Source: CAD feature listing. Evaluate the final solid. Frame: model axes, mm. Face numbers are marked on the shaded views. A direction names the side the tool comes from. Round coordinates to 2 decimals unless told otherwise and drop trailing zeros. Loops run counter-clockwise (first coordinate to the right, second up) from the corner with the lowest first, then second, coordinate; pieces in that order, holes last. Notation, with made-up numbers: (71.25, 12) -> (120.25, 12) arc R20 cw to (120.25, 51) -> close; hole circle Ø9 at (66, 28.5). An arc over 180 degrees is marked (long way). Return JSON: item names as keys, results as strings. Group by question number.
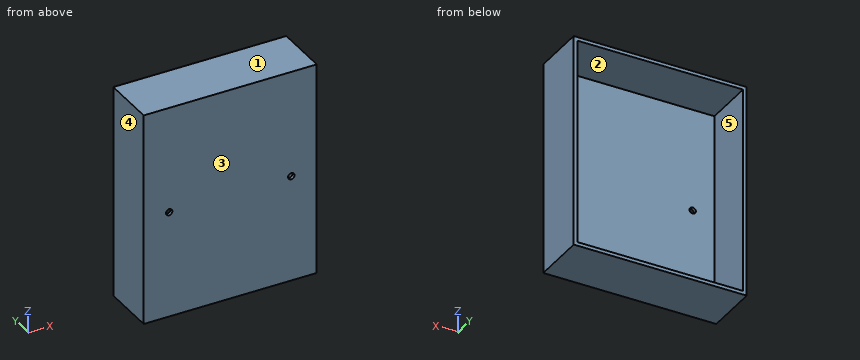
```python
from build123d import *

# Parameters (mm, degrees)
SKETCH1_W           = 61.2
SKETCH1_H           = 75.5
BOSS_EXTRUDE1_DEPTH = 19.15
SKETCH2_W           = 58.6
SKETCH2_H           = 72.89934915
CUT_EXTRUDE1_DEPTH  = 18
SKETCH3_R           = 1.125
CUT_EXTRUDE2_DEPTH  = 20


with BuildPart() as part:
    # Sketch1 → Boss-Extrude1 (new body)
    with BuildSketch(Plane(origin=(0, 0, 0), x_dir=(1, 0, 0), z_dir=(0, 1, 0))):
        Rectangle(SKETCH1_W, SKETCH1_H)
    extrude(amount=BOSS_EXTRUDE1_DEPTH)

    # Sketch2 → Cut-Extrude1 (cut)
    with BuildSketch(Plane(origin=(0, 19.15, 0), x_dir=(1, 0, 0), z_dir=(0, 1, 0))):
        Rectangle(SKETCH2_W, SKETCH2_H)
    extrude(amount=-CUT_EXTRUDE1_DEPTH, mode=Mode.SUBTRACT)

    # Sketch3 → Cut-Extrude2 (cut)
    with BuildSketch(Plane(origin=(0, 1.15, 0), x_dir=(1, 0, 0), z_dir=(0, 1, 0))):
        with Locations(Location((-21.6, 0, 0), (0, 0, 270))):
            Circle(SKETCH3_R)
        with Locations(Location((21.6, 0, 0), (0, 0, 270))):
            Circle(SKETCH3_R)
    extrude(amount=-CUT_EXTRUDE2_DEPTH, mode=Mode.SUBTRACT)


solid = part.part
```
(1) Cut plane B-B (z = 0). Return loops of the section in (x, y) (3 decimals).
(2) Pin query (flat end, axial travel): pin 1 (1 mm diameter, centred on x = -6, z = 28, fed in from +Y). Return the tip coordinate at first contact, or that it passes through.
(3) Mould query, pull axis X, two halves, no side actions, for the marked faces 3, 4 and 5. Classes: released by +X, released by -X, zero draft, split by the parting line, or undercut.
(4) Cut plane C-C (y = 11.5). Return loops of the section in (x, z), and give its area (3 significant figures).
(5) Cut plane A-A (x = -21.6). Return loops of the section in (y, z) (3 decimals), and give its area (3 significant figures).
(6) Set-up query: the marked faces 1 and 2. Return all of +Z, -Z, +X, -X, +Y, -Y with unobstructed straight access to the full face (end or side cutting, diameter ignored); none if empty.
(7) Cut plane D-D (z = -29). Return loops of the section in (x, y).
(8) Ray query, line 1 (X direction, y = 0.55, z = 0) (3 decimals); line 2 (Z direction, x = -5.5, y = 18); line 3 (X direction, y = 11.5, z = -0.5). Return the intervals inside material, ascending.
Answers follow:
{
 "1": {"outline": "(-30.6, 0) -> (-22.725, 0) -> (-22.725, 1.15) -> (-29.3, 1.15) -> (-29.3, 19.15) -> (-30.6, 19.15) -> close; (-20.475, 0) -> (20.475, 0) -> (20.475, 1.15) -> (-20.475, 1.15) -> close; (22.725, 0) -> (30.6, 0) -> (30.6, 19.15) -> (29.3, 19.15) -> (29.3, 1.15) -> (22.725, 1.15) -> close"},
 "2": {"pin 1": "y = 1.15"},
 "3": {"face 3": "zero draft", "face 4": "released by -X", "face 5": "undercut"},
 "4": {"outline": "(-30.6, -37.75) -> (30.6, -37.75) -> (30.6, 37.75) -> (-30.6, 37.75) -> close; hole (-29.3, -36.45) -> (29.3, -36.45) -> (29.3, 36.45) -> (-29.3, 36.45) -> close", "area": "349 mm^2"},
 "5": {"outline": "(0, -37.75) -> (19.15, -37.75) -> (19.15, -36.45) -> (1.15, -36.45) -> (1.15, -1.125) -> (0, -1.125) -> close; (0, 1.125) -> (1.15, 1.125) -> (1.15, 36.45) -> (19.15, 36.45) -> (19.15, 37.75) -> (0, 37.75) -> close", "area": "131 mm^2"},
 "6": {"face 1": "+Z, +X, -X, +Y, -Y", "face 2": "+Y"},
 "7": {"outline": "(-30.6, 0) -> (30.6, 0) -> (30.6, 19.15) -> (29.3, 19.15) -> (29.3, 1.15) -> (-29.3, 1.15) -> (-29.3, 19.15) -> (-30.6, 19.15) -> close"},
 "8": {"line 1": "-30.6 to -22.725, -20.475 to 20.475, 22.725 to 30.6", "line 2": "-37.75 to -36.45, 36.45 to 37.75", "line 3": "-30.6 to -29.3, 29.3 to 30.6"}
}
